Verification items for the finished model (mm, model axes). A direction names the side the tool comes from. Give positions to 0.01 mm unless a question says otherwise; leave off trailing zeros. Order: outer loops, then holes, each group sorted by start corner. A loop starts at its lowest first (then second) coordinate and runs counter-clockwise, first axis right, second up. Notation, with made-up numbers: (36, -26) -> (78, -26) arc R25 ccw to (78, 9) -> close; hole circle Ø7 at (-6.75, 7). An arc over 180 degrees is marked (long way). Write each question's results on one line, items separated by ' | '. Start each with the question number.
1. Cross-section at C-C, the plane z = 0. Enter the section's corners in (x, y).
2. Depth check by flat-ended pin: pin 1 Ø3 at (y, z) = (5, -23) entering from +X; pin 2 Ø0.8 at (x, y) = (0, 4) entering from -Z; pin 3 Ø3 at (x, y) = (13.5, 1) entering from +Z. Enter the tip coordinate at first touch or a pass-through.
3. Set-up check for faces 5 (the face through (3.5, 3, 23)), 6 (the face through (0, 4, -20.1)), 7 (the face through (3.5, 3, -23)), 8 (the face through (-3.5, 3, 23)), 9 (the face through (8.25, 7, 12.41)): record each of +Z, -Z, +X, -X, +Y, -Y from which the full face is reachable in a straight line by a thin tool's end or side.
4. Material ranges on L1, parallel to Y at x = 0, z = 21; L2, parallel to Z at x = 0, y = 7.75; L3, parallel to Y at x = -10, z = -20.5, recorded low to high. Write a range as from..to.
5. Mould release check, pull along Z, two halves, no side actions. Record for faces 1 (the face through (2, 3, 25.1)), 2 (the face through (14.07, 8.48, -4.43)), 3 (the face through (4.53, 10, 14.2)), 4 (the face through (-2.44, 3.45, -18.59)): +Z half, -Z half, draft (parallel to the pull), parting line (faces both ways), or undercut.
6. Cross-section at B-B, the plane z = 22.5. Enter the section's corners in (x, y), then the cut area to 3 significant figures.
7. Cross-section at A-A, the plane x = 0. Enter the section's corners in (y, z).
8. Cross-section at D-D, the plane x = -9.5. Enter the section's corners in (y, z), then the cut area to 3 significant figures.
from build123d import *

# Parameters (mm, degrees)
SKETCH1_R           = 18.75
BOSS_EXTRUDE1_DEPTH = 7
SKETCH2_R           = 1.5
CUT_EXTRUDE1_DEPTH  = 7
SKETCH3_R           = 1.4
CUT_EXTRUDE2_DEPTH  = 5
BOSS_EXTRUDE3_DEPTH = 7
SKETCH7_R           = 1.4
CUT_EXTRUDE3_DEPTH  = 7
SKETCH9_R           = 21.75
SKETCH9_R_2         = 14.75
BOSS_EXTRUDE5_DEPTH = 3


with BuildPart() as part:
    # Sketch1 → Boss-Extrude1 (new body)
    with BuildSketch(Plane(origin=(0, 0, 0), x_dir=(1, 0, 0), z_dir=(0, 1, 0))):
        with BuildLine():
            Line((3.5, -25.1), (-3.5, -25.1))
            Line((-3.5, -25.1), (-3.5, -21.466544))
            ThreePointArc((-3.5, -21.466544), (-21.75, 0), (-3.5, 21.466544))
            Line((-3.5, 21.466544), (-3.5, 25.1))
            Line((-3.5, 25.1), (3.5, 25.1))
            Line((3.5, 25.1), (3.5, 21.466544))
            ThreePointArc((3.5, 21.466544), (21.75, 0), (3.5, -21.466544))
            Line((3.5, -21.466544), (3.5, -25.1))
        make_face()
        Circle(SKETCH1_R, mode=Mode.SUBTRACT)
    extrude(amount=BOSS_EXTRUDE1_DEPTH)

    # Sketch2 → Cut-Extrude1 (cut)
    with BuildSketch(Plane.XY.offset(25.1)):
        with Locations((0, 3.5)):
            Circle(SKETCH2_R)
    extrude(amount=-CUT_EXTRUDE1_DEPTH, mode=Mode.SUBTRACT)

    # Sketch3 → Cut-Extrude2 (cut)
    with BuildSketch(Plane(origin=(0, 0, -25.1), x_dir=(-1, 0, 0), z_dir=(0, 0, -1))):
        with Locations((0, 3.5)):
            Circle(SKETCH3_R)
    extrude(amount=-CUT_EXTRUDE2_DEPTH, mode=Mode.SUBTRACT)

    # Sketch6 → Boss-Extrude3 (add)
    with BuildSketch(Plane(origin=(0, 0, 0), x_dir=(-1, 0, 0), z_dir=(0, -1, 0))):
        with BuildLine():
            Line((3.5, 25.1), (16.5, 25.1))
            Line((16.5, 25.1), (16.5, 14.170833))
            ThreePointArc((16.5, 14.170833), (10.644569, 18.967226), (3.5, 21.466544))
            Line((3.5, 21.466544), (3.5, 25.1))
        make_face()
    extrude(amount=-BOSS_EXTRUDE3_DEPTH)

    # Sketch7 → Cut-Extrude3 (cut)
    with BuildSketch(Plane(origin=(0, 0, -25.1), x_dir=(-1, 0, 0), z_dir=(0, 0, -1))):
        with Locations((10, 3.5)):
            Circle(SKETCH7_R)
    extrude(amount=-CUT_EXTRUDE3_DEPTH, mode=Mode.SUBTRACT)

    # Sketch9 → Boss-Extrude5 (add)
    with BuildSketch(Plane(origin=(0, 7, 0), x_dir=(1, 0, 0), z_dir=(0, 1, 0))):
        Circle(SKETCH9_R)
        Circle(SKETCH9_R_2, mode=Mode.SUBTRACT)
    extrude(amount=BOSS_EXTRUDE5_DEPTH)


solid = part.part
Results below:
1) outline: (-21.75, 0) -> (-18.75, 0) -> (-18.75, 7) -> (-14.75, 7) -> (-14.75, 10) -> (-21.75, 10) -> close; (14.75, 7) -> (18.75, 7) -> (18.75, 0) -> (21.75, 0) -> (21.75, 10) -> (14.75, 10) -> close
2) pin 1: stops at x = 3.5 | pin 2: stops at z = -20.1 | pin 3: stops at z = 18.14
3) face 5: +Z, +X, +Y, -Y | face 6: -Z | face 7: -Z, +X, +Y, -Y | face 8: +Z, -X, +Y, -Y | face 9: -Y
4) L1: y = 0..2, 5..10 | L2: z = -21.75..-14.75, 14.75..21.75 | L3: y = 0..2.1, 4.9..7
5) face 1: +Z half | face 2: undercut | face 3: draft | face 4: undercut
6) outline: (-3.5, 0) -> (3.5, 0) -> (3.5, 7) -> (-3.5, 7) -> close; hole circle Ø3 at (0, 3.5) | area: 41.9 mm²
7) outline: (0, -25.1) -> (2.1, -25.1) -> (2.1, -20.1) -> (4.9, -20.1) -> (4.9, -25.1) -> (7, -25.1) -> (7, -21.75) -> (10, -21.75) -> (10, -14.75) -> (7, -14.75) -> (7, -18.75) -> (0, -18.75) -> close; (0, 18.75) -> (2, 18.75) -> (2, 25.1) -> (0, 25.1) -> close; (5, 18.75) -> (7, 18.75) -> (7, 14.75) -> (10, 14.75) -> (10, 21.75) -> (7, 21.75) -> (7, 25.1) -> (5, 25.1) -> close
8) outline: (0, -25.1) -> (2.19, -25.1) -> (2.19, -18.1) -> (4.81, -18.1) -> (4.81, -25.1) -> (7, -25.1) -> (7, -19.57) -> (10, -19.57) -> (10, -11.28) -> (7, -11.28) -> (7, -16.17) -> (0, -16.17) -> close; (0, 16.17) -> (7, 16.17) -> (7, 11.28) -> (10, 11.28) -> (10, 19.57) -> (0, 19.57) -> close | area: 118 mm²
